from build123d import *

# Parameters (mm, degrees)
F1_DEPTH = 5.08
F2_R     = 1.5875
F3_DEPTH = 25.4
F4_R     = 2.54
F5_R     = 19.05
F6_DEPTH = 2.54


with BuildPart() as f1:
    # F0 (on Front) → F1 (new body)
    with BuildSketch(Plane.XZ):
        with BuildLine():
            ThreePointArc((0, 7.62), (2.231846, 2.231846), (7.62, 0))
            Line((7.62, 0), (36.83, 0))
            ThreePointArc((36.83, 0), (42.218154, 2.231846), (44.45, 7.62))
            Line((44.45, 7.62), (44.45, 49.53))
            ThreePointArc((44.45, 49.53), (42.218154, 54.918154), (36.83, 57.15))
            Line((36.83, 57.15), (7.62, 57.15))
            ThreePointArc((7.62, 57.15), (2.231846, 54.918154), (0, 49.53))
            Line((0, 49.53), (0, 7.62))
        make_face()
    extrude(amount=F1_DEPTH)

    # F2 (on Front) → F3 (cut)
    with BuildSketch(Plane.XZ):
        with Locations((22.225, 51.816)):
            Circle(F2_R)
        with Locations((22.225, 5.334)):
            Circle(F2_R)
    extrude(amount=F3_DEPTH, mode=Mode.SUBTRACT)

    # F4
    f4_edges = [f1.edges().sort_by_distance(p)[0] for p in [
        (22.225, -5.08, 57.15),
    ]]
    fillet(f4_edges, radius=F4_R)

    # F5 (on face) → F6 (cut)
    with BuildSketch(Plane.XZ.offset(5.08)):
        with Locations((22.225, 28.575)):
            Circle(F5_R)
    extrude(amount=-F6_DEPTH, mode=Mode.SUBTRACT)


solid = f1.part
Model file for the job. Use its own axes, mm. A direction names the side the tool comes from. Give positions to 0.01 mm unless a question says otherwise; leave off trailing zeros. Order: outer loops, then holes, each group sorted by start corner. A loop starts at its lowest first (then second) coordinate and runs counter-clockwise, first axis right, second up. Notation, with made-up numbers: M -19.5,80 L 37.5,80 A21 cw 37.5,112 Z; hole C 46,0 d3. An arc over 180 degrees is marked long. Write item = value, one per line.
Q1. Tool access for faces 5 (the cylindrical face through (22.021, -4.356, 56.386)), 6 (the cylindrical face through (18, -4, 10)): list every direction of +Z, -Z, +X, -X, +Y, -Y with a clear straight run to the whole face (end or side of a thin tool).
Derived:
face_5 = +Z, +X, -X, -Y
face_6 = -Y
Q2. Cut at D-D, the plane x = 33. List the corners of the cut face in (y, z).
Derived:
outline = M -5.08,2.54 A2.54 ccw -2.54,0 L 0,0 L 0,57.15 L -2.54,57.15 A2.54 ccw -5.08,54.61 L -5.08,44.28 L -2.54,44.28 L -2.54,12.87 L -5.08,12.87 Z
Q3. Cut at B-B, the plane x = 23. List the corners of the cut face in (y, z), then the cut area to 3 significant figures.
Derived:
outline = M -5.08,2.54 A2.54 ccw -2.54,0 L 0,0 L 0,3.95 L -5.08,3.95 Z; M -5.08,6.72 L 0,6.72 L 0,50.43 L -5.08,50.43 L -5.08,47.61 L -2.54,47.61 L -2.54,9.54 L -5.08,9.54 Z; M -5.08,53.2 L 0,53.2 L 0,57.15 L -2.54,57.15 A2.54 ccw -5.08,54.61 Z
area = 163 mm2
Q4. Cut at A-A, the plane y = -1.85. Count the separate pieces of the cut face and the enclosed holes in it, then the cut area to 3 significant figures.
Derived:
separate_pieces = 1
enclosed_holes = 2
area = 2,470 mm2
Q5. Two-plate mould, pull along X, no slides. Class faces 1 (the cylindrical face through (21.881, -2.504, 50.266)), 2 (the flat face through (22, -2.54, 29)), 3 (the flat face through (22, 0, 29)), 4 (the cylindrical face through (42.159, -1.252, 2.173)): pulls with the +X half, pulls with the -X half, needs draft (parallel to the pull), parting line crosses it, or undercut.
Derived:
face_1 = undercut
face_2 = undercut
face_3 = needs draft
face_4 = pulls with the +X half
Q6. Cut at C-C, the plane z = 45.5. List the corners of the cut face in (x, y).
Derived:
outline = M 0,-2.54 A2.54 ccw 2.54,-5.08 L 13.48,-5.08 L 13.48,-2.54 L 30.97,-2.54 L 30.97,-5.08 L 41.91,-5.08 A2.54 ccw 44.45,-2.54 L 44.45,0 L 0,0 Z
Q7. Drill centre lines: line 1 (Z direction, x = 21.5, y = -1.7); line 2 (Z direction, x = 21, y = -1.8); line 3 (Y direction, x = 15, z = 33.5). Where is each one in solid material? Low to high. Write a range as [from, to].
Derived:
line_1 = [0, 3.92], [6.75, 50.4], [53.23, 57.15]
line_2 = [0, 4.32], [6.34, 50.81], [52.83, 57.15]
line_3 = [-2.54, 0]
Q8. Flat gauge pins, fed straight in: pin 1 (19 mm diameter, centred on x = 25.5, z = 20, fed in from -Y); pin 2 (1 mm diameter, centred on y = -4.5, z = 12, fed in from +X). Where does each tip first touch, or does it go through?
Derived:
pin_1 = -2.54
pin_2 = 43.99
